Geometry check sheet. Reference: the model listing, model coordinates, mm. A direction names the side the tool comes from. Coordinates: 2 decimals unless noted, no trailing zeros. Write each loop counter-clockwise with the first axis right and the second up, starting at its lowest first coordinate (ties: lowest second). Pieces come first, ordered by that corner, then holes. Notation, with made-up numbers: (66, -17.5) -> (107, -17.5) arc R22 ccw to (107, -9.5) -> close; hole circle Ø1 at (64, -26.75). An arc over 180 degrees is marked (long way). Put each result on its own line as item: value. Start each with the question number.
from build123d import *

# Parameters (mm, degrees)
SKETCH1_R           = 2.159
SKETCH1_W           = 6.35
SKETCH1_H           = 6.35
BOSS_EXTRUDE1_DEPTH = 6.35


with BuildPart() as part:
    # Sketch1 → Boss-Extrude1 (new body)
    with BuildSketch(Plane(origin=(0, 0, 0), x_dir=(1, 0, 0), z_dir=(0, 1, 0))):
        Polygon((-57.15, 101.6), (-25.4, 101.6), (-25.4, 25.4), (-13.208, 25.4), (-13.208, 82.55), (-6.858, 82.55), (-6.858, 25.4), (6.858, 25.4), (6.858, 82.55), (13.208, 82.55), (13.208, 25.4), (25.4, 25.4), (25.4, 101.6), (57.15, 101.6), (57.15, -101.6), (-57.15, -101.6), align=None)
        with Locations(Location((34.925, 80.391, 0), (0, 0, 270))):
            Circle(SKETCH1_R, mode=Mode.SUBTRACT)
        with Locations(Location((-34.925, 80.391, 0), (0, 0, 270))):
            Circle(SKETCH1_R, mode=Mode.SUBTRACT)
        with Locations(Location((47.625, 80.391, 0), (0, 0, 270))):
            Circle(SKETCH1_R, mode=Mode.SUBTRACT)
        with Locations(Location((-47.625, 80.391, 0), (0, 0, 270))):
            Circle(SKETCH1_R, mode=Mode.SUBTRACT)
        with Locations(Location((47.625, -80.391, 0), (0, 0, 270))):
            Circle(SKETCH1_R, mode=Mode.SUBTRACT)
        with Locations(Location((-47.625, -80.391, 0), (0, 0, 270))):
            Circle(SKETCH1_R, mode=Mode.SUBTRACT)
        with Locations((34.925, 92.075)):
            Rectangle(SKETCH1_W, SKETCH1_H, mode=Mode.SUBTRACT)
        with Locations((34.925, 68.707)):
            Rectangle(SKETCH1_W, SKETCH1_H, mode=Mode.SUBTRACT)
        with Locations((-34.925, 92.075)):
            Rectangle(SKETCH1_W, SKETCH1_H, mode=Mode.SUBTRACT)
        with Locations((-34.925, 68.707)):
            Rectangle(SKETCH1_W, SKETCH1_H, mode=Mode.SUBTRACT)
        with Locations((47.625, 92.075)):
            Rectangle(SKETCH1_W, SKETCH1_H, mode=Mode.SUBTRACT)
        with Locations((47.625, 68.707)):
            Rectangle(SKETCH1_W, SKETCH1_H, mode=Mode.SUBTRACT)
        with Locations((-47.625, 92.075)):
            Rectangle(SKETCH1_W, SKETCH1_H, mode=Mode.SUBTRACT)
        with Locations((-47.625, 68.707)):
            Rectangle(SKETCH1_W, SKETCH1_H, mode=Mode.SUBTRACT)
        with Locations((47.625, -68.707)):
            Rectangle(SKETCH1_W, SKETCH1_H, mode=Mode.SUBTRACT)
        with Locations((47.625, -92.075)):
            Rectangle(SKETCH1_W, SKETCH1_H, mode=Mode.SUBTRACT)
        with Locations((-47.625, -68.707)):
            Rectangle(SKETCH1_W, SKETCH1_H, mode=Mode.SUBTRACT)
        with Locations((-47.625, -92.075)):
            Rectangle(SKETCH1_W, SKETCH1_H, mode=Mode.SUBTRACT)
    extrude(amount=BOSS_EXTRUDE1_DEPTH)


solid = part.part
Item 1: Section check D-D, the plane y = 1.5. Give the number of separate pieces and of enclosed holes in the cut face, and give its area (3 significant figures).
Item 2: Section check C-C, the plane x = -18.5. Enter the section's corners in (y, z).
Item 3: Section check B-B, the plane z = -35. Enter the section's corners in (x, y).
Item 4: Access from +Z, -Z, +X, -X, +Y, -Y to the whole of each face (thin tool, end or side, straight path). Record for faces 4 (the flat face through (25.4, 3, -63)), 5 (the flat face through (-48, 3, -65.532)).
Item 5: Section check A-A, the plane z = 70. Enter the section's corners in (x, y), and give its area (3 significant figures).
Item 6: Mould release check, pull along X, two halves, no side actions. Record for faces 1 (the flat face through (35, 3, -88.9)), 2 (the flat face through (-57.15, 3, 1)), 3 (the flat face through (-41, 3, -101.6)): released by +X, released by -X, zero draft, split by the parting line, or undercut.
Item 7: Go/stop test with flat-tipped pins: P1, Ø3, axis at x = 22.5, y = 4, coming from the -Z side; P2, Ø4, axis at x = -47.625, z = 80.391, coming from the +Y side. Record where each tip stops, or that it passes through.
Item 8: Scan lines: line 1 along X through (y, z) = (5.75, -53.5); line 2 along Z through (x, y) = (45, 2); line 3 along X through (y, z) = (3.5, 67.5). Record each from-to range of solid material in increasing order. Write a range as [from, to].
From the geometry:
1. separate pieces: 1
1. enclosed holes: 18
1. area: 19,500 mm²
2. outline: (0, -25.4) -> (6.35, -25.4) -> (6.35, 101.6) -> (0, 101.6) -> close
3. outline: (-57.15, 0) -> (-25.4, 0) -> (-25.4, 6.35) -> (-57.15, 6.35) -> close; (-13.21, 0) -> (-6.86, 0) -> (-6.86, 6.35) -> (-13.21, 6.35) -> close; (6.86, 0) -> (13.21, 0) -> (13.21, 6.35) -> (6.86, 6.35) -> close; (25.4, 0) -> (57.15, 0) -> (57.15, 6.35) -> (25.4, 6.35) -> close
4. face 4: -Z, +Y, -Y
4. face 5: +Y, -Y
5. outline: (-57.15, 0) -> (-50.8, 0) -> (-50.8, 6.35) -> (-57.15, 6.35) -> close; (-44.45, 0) -> (44.45, 0) -> (44.45, 6.35) -> (-44.45, 6.35) -> close; (50.8, 0) -> (57.15, 0) -> (57.15, 6.35) -> (50.8, 6.35) -> close
5. area: 645 mm²
6. face 1: undercut
6. face 2: released by -X
6. face 3: zero draft
7. P1: z = -25.4
7. P2: through
8. line 1: [-57.15, -25.4], [-13.21, -6.86], [6.86, 13.21], [25.4, 57.15]
8. line 2: [-101.6, -95.25], [-88.9, -71.88], [-65.53, 65.53], [71.88, 88.9], [95.25, 101.6]
8. line 3: [-57.15, -50.8], [-44.45, 44.45], [50.8, 57.15]
